Source: CAD feature listing. Evaluate the final solid. Frame: model axes, mm. Face numbers are marked on the shaded views. A direction names the side the tool comes from. Coordinates: 2 decimals unless noted, no trailing zeros. Order: outer loops, then holes, each group sorted by start corner. A loop starts at its lowest first (then second) coordinate and runs counter-clockwise, first axis right, second up.
Autodesk Inventor part; units mm, degrees
ref_plane "YZ Plane" through (0, 0, 0) normal (1, 0, 0) x (0, 1, 0)
ref_plane "XZ Plane" through (0, 0, 0) normal (0, 1, 0) x (-1, 0, 0)
ref_plane "XY Plane" through (0, 0, 0) normal (0, 0, 1) x (1, 0, 0)
sketch "Эскиз1" plane through (0, 0, 0) normal (0, 1, 0) x (-1, 0, 0)
  circle A0 centre (0, 0) radius 11
  dimension "d0" = 22
extrude "Выдавливание1" add sketch "Эскиз1" along normal blind 2
sketch "Эскиз2" plane through (0, 2, 0) normal (0, 1, 0) x (1, 0, 0)
  circle A0 centre (0, 0) radius 5
  dimension "d3" = 10
extrude "Выдавливание2" add sketch "Эскиз2" along normal blind 10
sketch "Эскиз3" plane through (0, 12, 0) normal (0, 1, 0) x (1, 0, 0)
  circle A0 centre (0, 0) radius 2.5
  dimension "d6" = 5
extrude "Выдавливание3" cut sketch "Эскиз3" against normal blind 12
sketch "Эскиз4" plane through (0, 2, 0) normal (0, 1, 0) x (1, 0, 0)
  circle A0 centre (0, 0) radius 8 construction
  circle A1 centre (-8, 0) radius 1.5
  circle A2 centre (0, -8) radius 1.5
  circle A3 centre (8, 0) radius 1.5
  circle A4 centre (0, 8) radius 1.5
  dimension "d9" = 16
  dimension "d10" = 3
  dimension "d13" = 360
extrude "Выдавливание4" cut sketch "Эскиз4" against normal blind 2
properties part number "муфта"
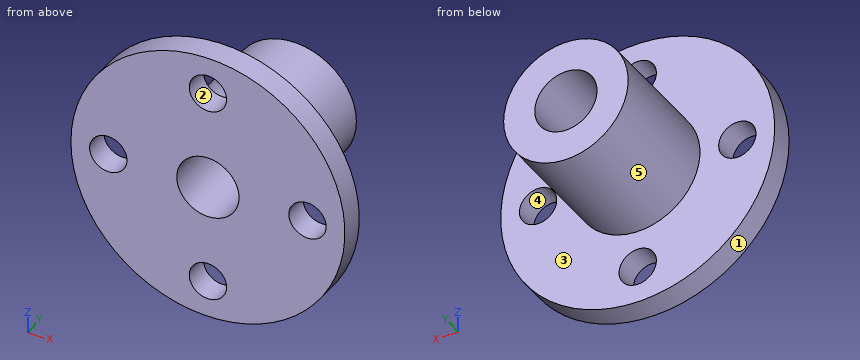
1. Pin query (flat end, axial travel): P1, Ø4, axis at x = 3.5, z = -7.5, coming from the +Y side; P2, Ø2.5, axis at x = -8, z = 0, coming from the -Y side; P3, Ø2, axis at y = 4.5, z = -4, coming from the +X side; P4, Ø5, axis at x = -6.5, y = 9.5, coming from the -Z side. Return the tip coordinate at first contact, or that it passes through.
Findings:
P1: stops at y = 2
P2: passes through
P3: stops at x = 4
P4: stops at z = -3
2. Draft query along Z for the marked faces 1, 2 and 3. Return one class per face: released by +Z, released by -Z, zero draft, split by the parting line, or undercut.
Findings:
face 1: split by the parting line
face 2: undercut
face 3: zero draft
3. Section query A-A on z = 0. Return loops of the section in (x, y), plus the area to 3 significant figures.
Findings:
outline: (-11, 0) - (-9.5, 0) - (-9.5, 2) - (-11, 2) - close; (-6.5, 0) - (-2.5, 0) - (-2.5, 12) - (-5, 12) - (-5, 2) - (-6.5, 2) - close; (2.5, 0) - (6.5, 0) - (6.5, 2) - (5, 2) - (5, 12) - (2.5, 12) - close; (9.5, 0) - (11, 0) - (11, 2) - (9.5, 2) - close
area: 72.0 mm2
4. Ray query, line 1 (Z direction, x = 0, y = 1.25); line 2 (Y direction, x = -9, z = -2.75); line 3 (Z direction, x = -0.25, y = 8.25). Return the intervals inside material, ascending.
Findings:
line 1: z = -11 to -9.5, -6.5 to -2.5, 2.5 to 6.5, 9.5 to 11
line 2: y = 0 to 2
line 3: z = -4.99 to -2.49, 2.49 to 4.99
5. Section query D-D on y = 2.75. Return loops of the section in (x, z), plus the area to 3 significant figures.
Findings:
outline: circle Ø10 at (0, 0); hole circle Ø5 at (0, 0)
area: 58.9 mm2
6. Access query for the marked faces 4 and 5. Directions: +Z, -Z, +X, -X, +Y, -Y. A direction counts if a zero-diameter tool reaches every point of the face in a straight line with its end or side. Return the directions, or none.
Findings:
face 4: +Y, -Y
face 5: +Y
7. Section query C-C on x = -9. Return loops of the section in (y, z).
Findings:
outline: (0, -6.32) - (2, -6.32) - (2, -1.12) - (0, -1.12) - close; (0, 1.12) - (2, 1.12) - (2, 6.32) - (0, 6.32) - close
8. Section query B-B on z = -8. Return loops of the section in (x, y).
Findings:
outline: (-7.55, 0) - (-1.5, 0) - (-1.5, 2) - (-7.55, 2) - close; (1.5, 0) - (7.55, 0) - (7.55, 2) - (1.5, 2) - close
